For this review, take the finished solid that the model builds, in its own axes (mm). Face numbers are marked on the shaded views. A direction names the side the tool comes from. Give positions to 0.01 mm unless a question says otherwise; leave off trailing zeros. Order: outer loops, then holes, each group sorted by start corner. A loop starts at its lowest first (then second) coordinate and runs counter-clockwise, first axis right, second up. Notation, with made-up numbers: (79, -9) -> (119, -9) arc R23 ccw to (119, 12) -> close; hole circle Ø1 at (25, 66.5). An arc over 180 degrees is marked (long way). Return JSON: item names as keys, results as strings. Group by question number.
1) Add section C-C (z = 3). Give the boundary of the cut face in (x, y) (1 decimal).
2) For the marked faces 1 and 2, list the 3-axis set-ups (+Z, -Z, +X, -X, +Y, -Y) from which the entire face can be reached by the end or side of a thin tool; tool diameter is ignored.
3) Insertion check: P1, Ø2, axis at x = 12, z = 10.5, coming from the +Y side; P2, Ø4, axis at y = -19, z = 6, coming from the -X side; P3, Ø0.7, axis at x = 11, y = -23.5, coming from the +Z side; P4, Ø0.7, axis at x = 11, y = -23.5, coming from the -Z side. Each pin has a flat end and moves straight along its axis. Give the tip position at first contact, or say it passes through.
4) Add section B-B (y = -13.5). Give the boundary of the cut face in (x, z), then the cut area to 3 significant figures.
5) To check wall thickness, follow line 1 along Z through (x, y) = (-10, 17); line 2 along Y through (x, z) = (-0.5, 4.5); line 3 along X through (y, z) = (-21, 8.5). State the ranges of each line that lie inside material, in increasing order.
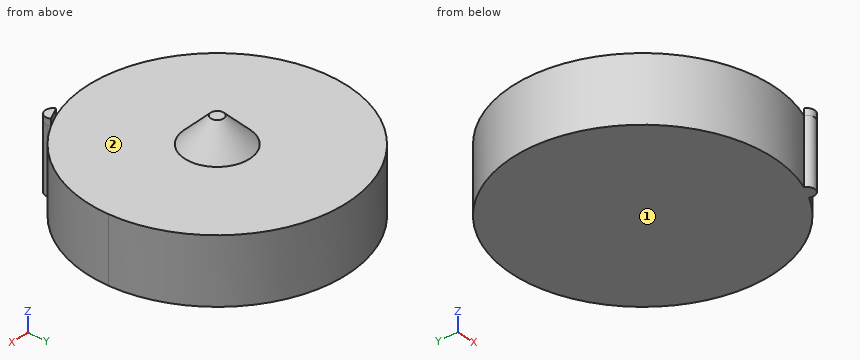
from build123d import *

# Parameters (mm, degrees)
F0_R     = 6.35
F1_DEPTH = 12.7
F2_DEPTH = 17.78
F3_SIZE  = 5.07999
F5_DEPTH = 1.27


# Not quite as in the source:
# - a fillet or chamfer is up to 0.001 mm smaller than in the source, because OpenCascade refuses the exact size


with BuildPart() as f1:
    # F0 (on Top) → F1 (new body)
    with BuildSketch(Plane.XY):
        with BuildLine():
            ThreePointArc((12.068946544, -22.3495084805), (21.8141151805, -13.011701614), (25.4, 0))
            ThreePointArc((25.4, 0), (-21.0057565892, 14.2799926511), (9.3434495971, -23.6190590335))
            ThreePointArc((9.3434495971, -23.6190590335), (10.0899459577, -21.6613011879), (12.068946544, -22.3495084805))
        make_face()
        Circle(F0_R, mode=Mode.SUBTRACT)
        with BuildLine():
            ThreePointArc((12.068946544, -22.3495084805), (10.0899459577, -21.6613011879), (9.3434495971, -23.6190590335))
            ThreePointArc((9.3434495971, -23.6190590335), (10.7249996167, -23.0246472986), (12.068946544, -22.3495084805))
        make_face()
        with BuildLine():
            ThreePointArc((12.068946544, -22.3495084805), (10.7249996167, -23.0246472986), (9.3434495971, -23.6190590335))
            ThreePointArc((9.3434495971, -23.6190590335), (11.0284458537, -24.4977142177), (12.2289962148, -23.0246472986))
            ThreePointArc((12.2289962148, -23.0246472986), (12.1884369016, -22.677722119), (12.068946544, -22.3495084805))
        make_face()
    extrude(amount=F1_DEPTH)

    # F0 (on Top) → F2 (join)
    with BuildSketch(Plane.XY):
        Circle(F0_R)
    extrude(amount=F2_DEPTH)

    # F3 (size 5.08 in the source; OpenCascade refuses exactly that, so slightly less here)
    f3_edges = [f1.edges().sort_by_distance(p)[0] for p in [
        (-6.35, 0, 17.78),
    ]]
    chamfer(f3_edges, length=F3_SIZE)

    # F4 (on face) → F5 (join)
    with BuildSketch(Plane.XY.offset(12.7)):
        with BuildLine():
            Line((12.068946544, -22.3495084805), (9.3434495971, -23.6190590335))
            ThreePointArc((9.3434495971, -23.6190590335), (11.3711055832, -24.4117207278), (12.068946544, -22.3495084805))
        make_face()
    extrude(amount=F5_DEPTH)


solid = f1.part
Evaluation:
{
 "1": {"outline": "(9.3, -23.6) arc R1.5 ccw (long way) to (12.1, -22.3) arc R25.4 ccw (long way) to start"},
 "2": {"face 1": "-Z, +X, -X, +Y, -Y", "face 2": "+Z"},
 "3": {"P1": "y = 22.89", "P2": "x = -18.87", "P3": "z = 13.97", "P4": "z = 0"},
 "4": {"outline": "(-21.52, 0) -> (21.52, 0) -> (21.52, 12.7) -> (-21.52, 12.7) -> close", "area": "546 mm^2"},
 "5": {"line 1": "0 to 12.7", "line 2": "-25.4 to 25.4", "line 3": "-14.29 to 14.29"}
}
